Design review of the part built by this model. Coordinates are the model's own, in mm. A direction names the side the tool comes from. Give positions to 0.01 mm unless a question says otherwise; leave off trailing zeros. Write each loop counter-clockwise with the first axis right and the second up, starting at its lowest first coordinate (ties: lowest second). Pieces come first, ordered by that corner, then holes. Notation, with made-up numbers: (18.25, 66) -> (73.25, 66) arc R6 cw to (73.25, 75) -> close; hole circle Ø3 at (-26, -21.75). An arc over 180 degrees is marked (long way). Return JSON: item names as keys, results as strings. Group by question number.
from build123d import *

# Parameters (mm, degrees)
SKETCH4_W                       = 106
SKETCH4_H                       = 16
BOSS_EXTRUDE2_DEPTH             = 13
CUT_EXTRUDE3_START              = -9.7
SKETCH25_W                      = 106
SKETCH25_H                      = 8.1
CUT_EXTRUDE3_DEPTH              = 107.216438698
M3X0_5_TAPPED_HOLE1_D           = 2.5
MIRROR1_START                   = -24.601316976
MIRROR1_OUTLINE_W               = 106
MIRROR1_OUTLINE_H               = 13
MIRROR1_OUTLINE_R               = 1.25
MIRROR1_DEPTH                   = 7.951316976
MIRROR1_START_2                 = -32.65
MIRROR1_2_OUTLINE_W             = 106
MIRROR1_2_OUTLINE_H             = 3.3
MIRROR1_2_DEPTH                 = 8.048683024
F_4_40_TAPPED_HOLE1_D           = 2.2606
F_4_40_TAPPED_HOLE1_ON_FACE_2_D = 2.2606


# Read off the part's stored shape, not the designer's step: Mirror1
with BuildPart() as part:
    # Sketch4 → Boss-Extrude2 (new body)
    with BuildSketch(Plane.XY):
        with Locations((-36.891047602, -24.65)):
            Rectangle(SKETCH4_W, SKETCH4_H)
    extrude(amount=-BOSS_EXTRUDE2_DEPTH)

    # Sketch25 → Cut-Extrude3 (cut)
    with BuildSketch(Plane.XY.offset(CUT_EXTRUDE3_START)):
        with Locations((-36.891047602, -28.651316976)):
            Rectangle(SKETCH25_W, SKETCH25_H)
    extrude(amount=CUT_EXTRUDE3_DEPTH, mode=Mode.SUBTRACT)

    # M3x0.5 Tapped Hole1 (through all)
    with Locations(Plane(origin=(-74.391047602, -16.65, -5.55), x_dir=(0, 0, 1), z_dir=(0, 1, 0))):
        with Locations((0, 0), (0, 25), (0, 75), (0, 50)):
            Hole(M3X0_5_TAPPED_HOLE1_D / 2)

    # Mirror1 outline → Mirror1 (add)
    with BuildSketch(Plane(origin=(0, 0, 0), x_dir=(1, 0, 0), z_dir=(0, 1, 0)).offset(MIRROR1_START)):
        with Locations((-36.891047602, 19.5)):
            Rectangle(MIRROR1_OUTLINE_W, MIRROR1_OUTLINE_H)
        with Locations((-74.391047602, 20.45)):
            Circle(MIRROR1_OUTLINE_R, mode=Mode.SUBTRACT)
        with Locations((-49.391047602, 20.45)):
            Circle(MIRROR1_OUTLINE_R, mode=Mode.SUBTRACT)
        with Locations((-24.391047602, 20.45)):
            Circle(MIRROR1_OUTLINE_R, mode=Mode.SUBTRACT)
        with Locations((0.608952398, 20.45)):
            Circle(MIRROR1_OUTLINE_R, mode=Mode.SUBTRACT)
    extrude(amount=MIRROR1_DEPTH)

    # Mirror1 2 outline → Mirror1 2 (add)
    with BuildSketch(Plane(origin=(0, 0, 0), x_dir=(1, 0, 0), z_dir=(0, 1, 0)).offset(MIRROR1_START_2)):
        with Locations((-36.891047602, 14.65)):
            Rectangle(MIRROR1_2_OUTLINE_W, MIRROR1_2_OUTLINE_H)
    extrude(amount=MIRROR1_2_DEPTH)

    # #4-40 Tapped Hole1 (through all)
    with Locations(Plane(origin=(-83.891047602, -32.65, -12.801414568), x_dir=(0, 0, -1), z_dir=(0, -1, 0))):
        with Locations((0, 0), (0.13677014, 94), (0.355392609, 47)):
            Hole(F_4_40_TAPPED_HOLE1_D / 2)

    # #4-40 Tapped Hole1 on face 2 (through all)
    with Locations(Plane(origin=(-13.707536503, 0, 46.33240541), x_dir=(0, 0, -1), z_dir=(0, -1, 0))):
        with Locations((0, 0)):
            Hole(F_4_40_TAPPED_HOLE1_ON_FACE_2_D / 2)


solid = part.part
Q1. Take a section at B-B, the plane x = 6.5. Give the boundary of the cut face in (y, z), plus the area to 3 significant figures.
Q2. For L1, parallel to X at y = -19.5, z = -5.55; L2, parallel to X at y = -25, z = -13; L3, parallel to Z at x = 10, y = -22, list the stretches that pass through material, from the lowest coordinate up. Write a range as from..to.
Q3. Take a section at A-A, the plane z = -20.45. Give the boundary of the cut face in (x, y), plus the area to 3 significant figures.
Q4. Insertion check: pin 1 (8 mm diameter, centred on x = -35.5, z = -22, fed in from -Y); pin 2 (6.5 mm diameter, centred on x = -22.5, y = -29.5, fed in from +Z); pin 3 (6.5 mm diameter, centred on x = -56.5, y = -30, fed in from -Z). Each pin has a flat end and moves straight along its axis. Give the tip position at first contact, or say it passes through.
Q5. Take a section at C-C, the plane y = -20. Count the separate pieces of the cut face and the enclosed holes in it, plus the area to 3 significant figures.
Q6. Take a section at D-D, the plane z = -8. Give the boundary of the cut face in (x, y), plus the area to 3 significant figures.
Q7. Mouldability with a two-part tool opening along Z and no side actions: class faces 4 (the face through (-38, -24.601, -21)), 5 (the face through (-50.61, -20.68, -5.28)), 6 (the face through (-38, -21, -26)) as +Z half, -Z half, draft (parallel to the pull), parting line (faces both ways), or undercut.
Q8. Tool access review of faces 1 (the face through (-25.64, -20.68, -20.5)), 2 (the face through (-38, -24.601, -5)), 3 (the face through (-38, -29, -16.3)): name each direction out of +Z, -Z, +X, -X, +Y, -Y from which nothing blocks a thin tool from reaching the whole face with its end or side.
Final values:
{
 "1": {"outline": "(-32.65, -16.3) -> (-24.6, -16.3) -> (-24.6, -26) -> (-16.65, -26) -> (-16.65, 0) -> (-24.6, 0) -> (-24.6, -9.7) -> (-32.65, -9.7) -> close", "area": "260 mm²"},
 "2": {"L1": "x = -89.89..-75.64, -73.14..-50.64, -48.14..-25.64, -23.14..-0.64, 1.86..16.11", "L2": "x = -89.89..-85, -82.78..-38.01, -35.77..8.98, 11.24..16.11", "L3": "z = -26..-14.06, -11.81..0"},
 "3": {"outline": "(-89.89, -24.6) -> (-75.64, -24.6) -> (-75.64, -16.65) -> (-89.89, -16.65) -> close; (-73.14, -24.6) -> (-50.64, -24.6) -> (-50.64, -16.65) -> (-73.14, -16.65) -> close; (-48.14, -24.6) -> (-25.64, -24.6) -> (-25.64, -16.65) -> (-48.14, -16.65) -> close; (-23.14, -24.6) -> (-0.64, -24.6) -> (-0.64, -16.65) -> (-23.14, -16.65) -> close; (1.86, -24.6) -> (16.11, -24.6) -> (16.11, -16.65) -> (1.86, -16.65) -> close", "area": "763 mm²"},
 "4": {"pin 1": "stops at y = -24.6", "pin 2": "stops at z = -9.7", "pin 3": "stops at z = -16.3"},
 "5": {"separate pieces": "1", "enclosed holes": "11", "area": "2,700 mm²"},
 "6": {"outline": "(-89.89, -24.6) -> (16.11, -24.6) -> (16.11, -16.65) -> (-89.89, -16.65) -> close", "area": "843 mm²"},
 "7": {"face 4": "draft", "face 5": "undercut", "face 6": "-Z half"},
 "8": {"face 1": "+Y, -Y", "face 2": "+Z, +X, -X, -Y", "face 3": "-Z, +X, -X, -Y"}
}
